For this review, use the dimensioned drawing (mm, ordinates from the lowest corner) and the shaded views. Coordinates: 2 decimals unless noted, no trailing zeros. Order: outer loops, then holes, each group sorted by start corner. A loop starts at its lowest first (then second) coordinate and runs counter-clockwise, first axis right, second up. Notation, with made-up numbers: (3.25, 67) -> (10.25, 67) arc R18 cw to (10.25, 99) -> close; hole circle Ø5 at (51.5, -14.75). An arc over 180 degrees is marked (long way). Return JSON: item names as keys, results as strings. Group by question number.
Item 1: Take a section at C-C (x = 2.5). Write out the cut boundary in (y, z).
Item 2: Insertion check: pin 1 (8 mm diameter, centred on y = 8.5, z = 4, fed in from +X); pin 2 (1 mm diameter, centred on x = 8.5, z = 13.5, fed in from -Y); pin 3 (6 mm diameter, centred on x = 22.5, z = 16.5, fed in from -Y). Each pin has a flat end and moves straight along its axis. Give the tip position at first contact, or say it passes through.
Item 3: Draft analysis for pull direction Y (two halves, no side actions). For the marked faces 1, 2 and 3, state which applies: +Y half, -Y half, draft (parallel to the pull), parting line (faces both ways), or undercut.
Item 4: Take a section at B-B (y = 26). Write out the cut boundary in (x, z) (1 decimal).
Item 5: For line 1 along X through (y, z) = (12.5, 14.25); line 2 along Y through (x, z) = (3, 10) (1 decimal); line 3 along X through (y, z) = (3.5, 6) (1 decimal), list the stretches that pass through material, from the lowest coordinate up.
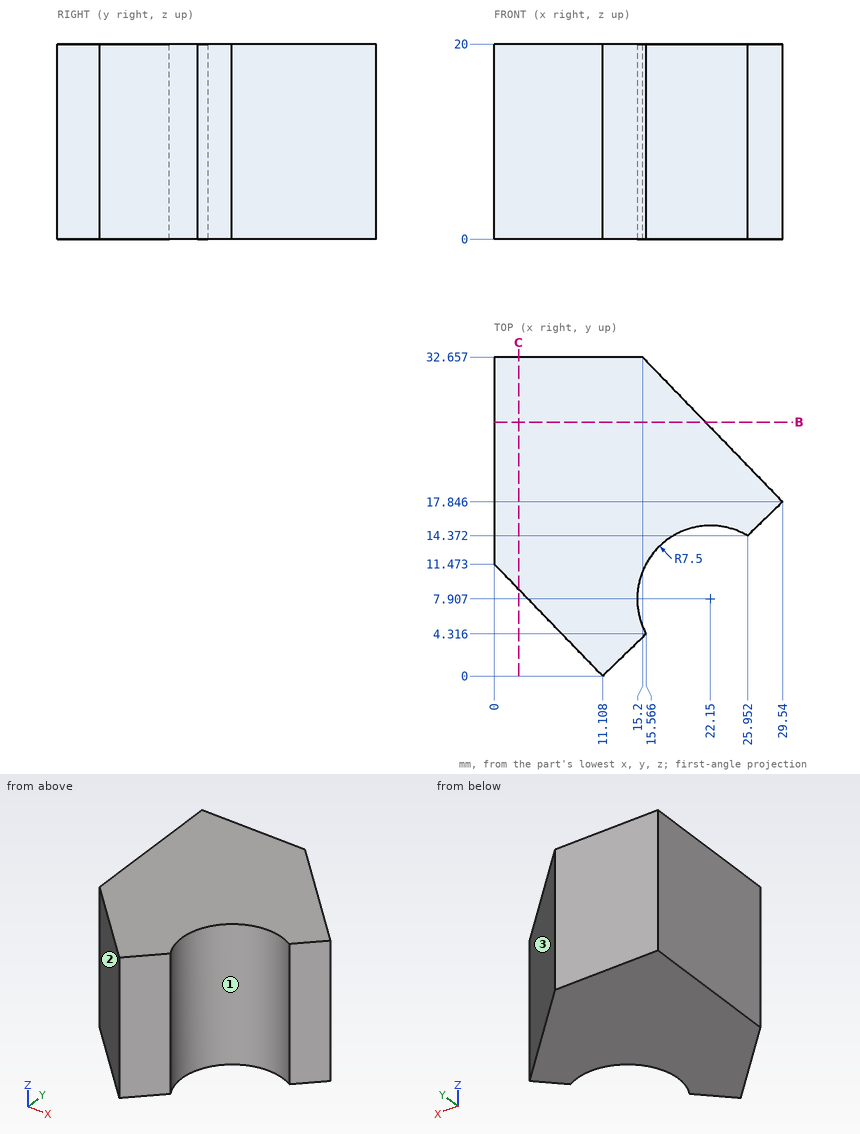
Findings below:
{
 "1": {"outline": "(8.89, 0) -> (32.66, 0) -> (32.66, 20) -> (8.89, 20) -> close"},
 "2": {"pin 1": "stops at x = 16.22", "pin 2": "stops at y = 2.18", "pin 3": "stops at y = 14.62"},
 "3": {"face 1": "undercut", "face 2": "-Y half", "face 3": "+Y half"},
 "4": {"outline": "(0, 0) -> (21.6, 0) -> (21.6, 20) -> (0, 20) -> close"},
 "5": {"line 1": "x = 0 to 16.22", "line 2": "y = 8.4 to 32.7", "line 3": "x = 7.7 to 14.7"}
}
